```python
from build123d import *

# Parameters (mm, degrees)
BOSS_EXTRUDE1_DEPTH = 15
CUT_EXTRUDE1_DEPTH  = 12
FILLET1_R           = 3
FILLET2_R           = 1.5
SKETCH6_R           = 1
CUT_EXTRUDE5_DEPTH  = 1
CUT_EXTRUDE6_DEPTH  = 2
SKETCH9_R           = 1.25
CUT_EXTRUDE7_DEPTH  = 3
SKETCH10_R          = 2.75
CUT_EXTRUDE8_DEPTH  = 1


with BuildPart() as part:
    # Sketch1 → Boss-Extrude1 (new body)
    with BuildSketch(Plane(origin=(0, 0, 0), x_dir=(1, 0, 0), z_dir=(0, 1, 0))):
        with BuildLine():
            Line((4, 0), (39, 0))
            ThreePointArc((39, 0), (41.828427125, 1.171572875), (43, 4))
            Line((43, 4), (43, 26))
            ThreePointArc((43, 26), (41.828427125, 28.828427125), (39, 30))
            Line((39, 30), (4, 30))
            ThreePointArc((4, 30), (1.171572875, 28.828427125), (0, 26))
            Line((0, 26), (0, 4))
            ThreePointArc((0, 4), (1.171572875, 1.171572875), (4, 0))
        make_face()
    extrude(amount=BOSS_EXTRUDE1_DEPTH)

    # Sketch2 → Cut-Extrude1 (cut)
    with BuildSketch(Plane.XZ):
        with BuildLine():
            Line((4, -2), (39, -2))
            ThreePointArc((39, -2), (40.414213562, -2.585786438), (41, -4))
            Line((41, -4), (41, -26))
            ThreePointArc((41, -26), (40.414213562, -27.414213562), (39, -28))
            Line((39, -28), (4, -28))
            ThreePointArc((4, -28), (2.585786438, -27.414213562), (2, -26))
            Line((2, -26), (2, -4))
            ThreePointArc((2, -4), (2.585786438, -2.585786438), (4, -2))
        make_face()
    extrude(amount=-CUT_EXTRUDE1_DEPTH, mode=Mode.SUBTRACT)

    # Fillet1
    fillet1_edges = [part.edges().sort_by_distance(p)[0] for p in [
        (1.171572875, 15, -28.828427125),
        (0, 15, -15),
        (1.171572875, 15, -1.171572875),
        (21.5, 15, 0),
        (41.828427125, 15, -1.171572875),
        (43, 15, -15),
        (41.828427125, 15, -28.828427125),
        (21.5, 15, -30),
    ]]
    fillet(fillet1_edges, radius=FILLET1_R)

    # Fillet2
    fillet2_edges = [part.edges().sort_by_distance(p)[0] for p in [
        (40.414213562, 12, -27.414213562),
        (21.5, 12, -28),
        (2.585786438, 12, -27.414213562),
        (2, 12, -15),
        (2.585786438, 12, -2.585786438),
        (21.5, 12, -2),
        (40.414213562, 12, -2.585786438),
        (41, 12, -15),
    ]]
    fillet(fillet2_edges, radius=FILLET2_R)

    # Sketch6 → Cut-Extrude5 (cut)
    with BuildSketch(Plane(origin=(0, 15, 0), x_dir=(1, 0, 0), z_dir=(0, 1, 0))):
        with BuildLine():
            Line((24.365034556, 14.814527437), (24.365034556, 7.958125892))
            Line((24.365034556, 7.958125892), (25.632801509, 9.225892845))
            ThreePointArc((25.632801509, 9.225892845), (26.33990829, 9.225892845), (26.33990829, 8.518786064))
            Line((26.33990829, 8.518786064), (24.218587947, 6.39746572))
            ThreePointArc((24.218587947, 6.39746572), (23.865034556, 6.251019111), (23.511481165, 6.39746572))
            Line((23.511481165, 6.39746572), (21.390160822, 8.518786064))
            ThreePointArc((21.390160822, 8.518786064), (21.390160822, 9.225892845), (22.097267603, 9.225892845))
            Line((22.097267603, 9.225892845), (23.365034556, 7.958125892))
            Line((23.365034556, 7.958125892), (23.365034556, 14.814527437))
            ThreePointArc((23.365034556, 14.814527437), (22.450820994, 15.336805548), (21.928542883, 16.251019111))
            Line((21.928542883, 16.251019111), (15.072141337, 16.251019111))
            Line((15.072141337, 16.251019111), (16.33990829, 14.983252158))
            ThreePointArc((16.33990829, 14.983252158), (16.33990829, 14.276145376), (15.632801509, 14.276145376))
            Line((15.632801509, 14.276145376), (13.511481165, 16.39746572))
            ThreePointArc((13.511481165, 16.39746572), (13.365034556, 16.751019111), (13.511481165, 17.104572501))
            Line((13.511481165, 17.104572501), (15.632801509, 19.225892845))
            ThreePointArc((15.632801509, 19.225892845), (16.33990829, 19.225892845), (16.33990829, 18.518786064))
            Line((16.33990829, 18.518786064), (15.072141337, 17.251019111))
            Line((15.072141337, 17.251019111), (21.928542883, 17.251019111))
            ThreePointArc((21.928542883, 17.251019111), (25.279248118, 18.165232673), (24.365034556, 14.814527437))
        make_face()
        with Locations((23.865034556, 16.751019111)):
            Circle(SKETCH6_R, mode=Mode.SUBTRACT)
        with BuildLine():
            Line((26.35894309, 18.994625435), (26.35894309, 23.705411504))
            ThreePointArc((26.35894309, 23.705411504), (25.85894309, 24.205411504), (25.35894309, 23.705411504))
            Line((25.35894309, 23.705411504), (25.35894309, 21.408838997))
            Line((25.35894309, 21.408838997), (22.176962575, 24.590819512))
            Line((22.176962575, 24.590819512), (22.176962575, 19.883712731))
            ThreePointArc((22.176962575, 19.883712731), (22.676962575, 19.383712731), (23.176962575, 19.883712731))
            Line((23.176962575, 19.883712731), (23.176962575, 22.17660595))
            Line((23.176962575, 22.17660595), (26.35894309, 18.994625435))
        make_face()
        with BuildLine():
            Line((28.940475029, 7.935307593), (31.233368247, 7.935307593))
            ThreePointArc((31.233368247, 7.935307593), (31.733368247, 8.435307593), (31.233368247, 8.935307593))
            Line((31.233368247, 8.935307593), (28.940475029, 8.935307593))
            Line((28.940475029, 8.935307593), (27.319154685, 10.556627936))
            ThreePointArc((27.319154685, 10.556627936), (26.612047904, 10.556627936), (26.612047904, 9.849521155))
            Line((26.612047904, 9.849521155), (28.026261466, 8.435307593))
            Line((28.026261466, 8.435307593), (26.612047904, 7.02109403))
            ThreePointArc((26.612047904, 7.02109403), (26.612047904, 6.313987249), (27.319154685, 6.313987249))
            Line((27.319154685, 6.313987249), (28.940475029, 7.935307593))
        make_face()
        with BuildLine():
            Line((10.334787343, 15.870919893), (11.749000906, 14.456706331))
            ThreePointArc((11.749000906, 14.456706331), (12.456107687, 14.456706331), (12.456107687, 15.163813112))
            Line((12.456107687, 15.163813112), (11.041894124, 16.578026674))
            Line((11.041894124, 16.578026674), (12.456107687, 17.992240237))
            ThreePointArc((12.456107687, 17.992240237), (12.456107687, 18.699347018), (11.749000906, 18.699347018))
            Line((11.749000906, 18.699347018), (10.334787343, 17.285133456))
            Line((10.334787343, 17.285133456), (8.920573781, 18.699347018))
            ThreePointArc((8.920573781, 18.699347018), (8.213467, 18.699347018), (8.213467, 17.992240237))
            Line((8.213467, 17.992240237), (9.627680562, 16.578026674))
            Line((9.627680562, 16.578026674), (8.213467, 15.163813112))
            ThreePointArc((8.213467, 15.163813112), (8.213467, 14.456706331), (8.920573781, 14.456706331))
            Line((8.920573781, 14.456706331), (10.334787343, 15.870919893))
        make_face()
    extrude(amount=-CUT_EXTRUDE5_DEPTH, mode=Mode.SUBTRACT)

    # Sketch7 → Cut-Extrude6 (cut)
    with BuildSketch(Plane.XY):
        with BuildLine():
            Line((19, 0), (24, 0))
            Line((24, 0), (24, 1))
            ThreePointArc((24, 1), (23.853553391, 1.353553391), (23.5, 1.5))
            Line((23.5, 1.5), (19.5, 1.5))
            ThreePointArc((19.5, 1.5), (19.146446609, 1.353553391), (19, 1))
            Line((19, 1), (19, 0))
        make_face()
    extrude(amount=-CUT_EXTRUDE6_DEPTH, mode=Mode.SUBTRACT)

    # Sketch9 → Cut-Extrude7 (cut)
    with BuildSketch(Plane(origin=(0, 15, 0), x_dir=(1, 0, 0), z_dir=(0, 1, 0))):
        with Locations((7, 7)):
            Circle(SKETCH9_R)
        with Locations((11.34, 22.96)):
            Circle(SKETCH9_R)
        with Locations((31.66, 22.96)):
            Circle(SKETCH9_R)
        with Locations((36, 7)):
            Circle(SKETCH9_R)
    extrude(amount=-CUT_EXTRUDE7_DEPTH, mode=Mode.SUBTRACT)

    # Sketch10 → Cut-Extrude8 (cut)
    with BuildSketch(Plane(origin=(0, 15, 0), x_dir=(1, 0, 0), z_dir=(0, 1, 0))):
        with Locations((7, 7)):
            Circle(SKETCH10_R)
        with Locations((11.34, 22.96)):
            Circle(SKETCH10_R)
        with Locations((36, 7)):
            Circle(SKETCH10_R)
        with Locations((31.66, 22.96)):
            Circle(SKETCH10_R)
    extrude(amount=-CUT_EXTRUDE8_DEPTH, mode=Mode.SUBTRACT)


solid = part.part
```
Geometry check sheet. Reference: the model listing, model coordinates, mm. A direction names the side the tool comes from. Coordinates: 2 decimals unless noted, no trailing zeros. Loops run counter-clockwise (first coordinate to the right, second up) from the corner with the lowest first, then second, coordinate; pieces in that order, holes last.
Item 1: Access from +Z, -Z, +X, -X, +Y, -Y to the whole of each face (thin tool, end or side, straight path). Record for faces 3 (the face through (24, 0.5, -1)), 4 (the face through (30.1, 14.5, -7.935)), 5 (the face through (21, 5, -2)).
Item 2: Sectioned sample at C-C, the plane x = 17. Record the boundary of the cut face in (y, z), then the cut area to 3 significant figures.
Item 3: Thickness scan on line 1 (Z direction, x = 6, y = 2); line 2 (X direction, y = 12.6, z = -7); line 3 (X direction, y = 14.7, z = -7). Record the ranges inside material, lowest first.
Item 4: Sectioned sample at A-A, the plane y = 6.5. Record the boundary of the cut face in (x, z).
Item 5: Sectioned sample at D-D, the plane z = -22.96. Count the separate pieces of the cut face and the enclosed holes in it, then the cut area to 3 significant figures.
Item 6: Go/stop test with flat-tipped pins: pin 1 Ø4 at (y, z) = (13, -16) entering from +X; pin 2 Ø1.6 at (x, z) = (32.5, -23) entering from +Y; pin 3 Ø0.8 at (y, z) = (14.5, -11) entering from +X; pin 4 Ø1.1 at (y, z) = (14.5, -22.5) entering from +X. Record where each tip stops, or that it passes through.
Item 7: Release check for a two-part mould opening along X. For faces 1 (the face through (24, 15, -17)), 2 (the face through (16.332, 14.507, -19.234)) record: released by +X, released by -X, zero draft, split by the parting line, or undercut.
Item 8: Sectioned sample at B-B, the plane x = 7. Record the boundary of the cut face in (y, z).
Check result:
1. face 3: +Z, -Y
1. face 4: +Y
1. face 5: -Y
2. outline: (0, -30) - (12, -30) arc R3 ccw to (15, -27) - (15, -17.25) - (14, -17.25) - (14, -16.25) - (15, -16.25) - (15, -3) arc R3 ccw to (12, 0) - (0, 0) - (0, -2) - (10.5, -2) arc R1.5 cw to (12, -3.5) - (12, -26.5) arc R1.5 cw to (10.5, -28) - (0, -28) - close
2. area: 134 mm2
3. line 1: z = -30 to -28, -2 to 0
3. line 2: x = 0.06 to 5.75, 8.25 to 34.75, 37.25 to 42.94
3. line 3: x = 1.69 to 4.25, 9.75 to 22.91, 24.82 to 26.59, 28.01 to 33.25, 38.75 to 41.31
4. outline: (0, -26) arc R4 ccw to (4, -30) - (39, -30) arc R4 ccw to (43, -26) - (43, -4) arc R4 ccw to (39, 0) - (4, 0) arc R4 ccw to (0, -4) - close; hole (2, -26) arc R2 ccw to (4, -28) - (39, -28) arc R2 ccw to (41, -26) - (41, -4) arc R2 ccw to (39, -2) - (4, -2) arc R2 ccw to (2, -4) - close
5. separate pieces: 3
5. enclosed holes: 0
5. area: 150 mm2
6. pin 1: stops at x = 43
6. pin 2: stops at y = 14
6. pin 3: stops at x = 42.14
6. pin 4: stops at x = 42.28
7. face 1: zero draft
7. face 2: undercut
8. outline: (0, -30) - (12, -30) arc R3 ccw to (15, -27) - (15, -9.75) - (14, -9.75) - (14, -8.25) - (12, -8.25) - (12, -26.5) arc R1.5 cw to (10.5, -28) - (0, -28) - close; (0, -2) - (10.5, -2) arc R1.5 cw to (12, -3.5) - (12, -5.75) - (14, -5.75) - (14, -4.25) - (15, -4.25) - (15, -3) arc R3 ccw to (12, 0) - (0, 0) - close
